```python
from build123d import *

# Parameters (mm, degrees)
PAD_DEPTH       = 15
PAD001_DEPTH    = 15
SKETCH002_R     = 4
POCKET_DEPTH    = 30
POCKET001_DEPTH = 4
SKETCH004_W     = 15
SKETCH004_H     = 50
PAD002_DEPTH    = 40
PAD003_DEPTH    = 50
SKETCH006_W     = 20
SKETCH006_H     = 5
POCKET002_DEPTH = 15
SKETCH007_W     = 30
SKETCH007_H     = 7.2
POCKET003_DEPTH = 3
SKETCH008_W     = 173.297394
SKETCH008_H     = 63.43742
POCKET004_DEPTH = 100
SKETCH009_W     = 20
SKETCH009_H     = 30
PAD004_DEPTH    = 15
SKETCH010_W     = 15
SKETCH010_H     = 30
PAD005_DEPTH    = 60
SKETCH011_R     = 2.5
POCKET005_DEPTH = 15
PAD006_DEPTH    = 30
SKETCH013_W     = 15
SKETCH013_H     = 20
POCKET006_DEPTH = 30
SKETCH014_R     = 2.5
POCKET007_DEPTH = 15
SKETCH015_R     = 6.7
POCKET008_DEPTH = 15
POCKET009_DEPTH = 4
SKETCH017_R     = 5.75
SKETCH017_R_2   = 4
PAD007_DEPTH    = 4
PAD008_DEPTH    = 15
SKETCH019_W     = 30
SKETCH019_H     = 12.5
POCKET010_DEPTH = 15
SKETCH020_R     = 2.5
POCKET011_DEPTH = 15


with BuildPart() as part:
    # Sketch → Pad (new body)
    with BuildSketch(Plane.XY):
        with BuildLine():
            ThreePointArc((6.422616, 1), (-6.5, 0), (6.422616, -1))
            Line((6.422616, -1), (20, -1))
            Line((20, -1), (20, -15))
            Line((20, -15), (-15, -15))
            Line((-15, -15), (-15, -7.5))
            Line((-30, -7.5), (-15, -7.5))
            Line((-45, -22.5), (-30, -7.5))
            Line((-45, -22.5), (-45, -45))
            Line((-180, -45), (-45, -45))
            Line((-180, 45), (-180, -45))
            Line((-180, 45), (-45, 45))
            Line((-45, 22.5), (-45, 45))
            Line((-45, 22.5), (-30, 7.5))
            Line((-30, 7.5), (-15, 7.5))
            Line((-15, 7.5), (-15, 15))
            Line((-15, 15), (20, 15))
            Line((20, 15), (20, 1))
            Line((6.422616, 1), (20, 1))
        make_face()
        Polygon((-60, 30), (-60, 2.330407), (-60, -7.217157), (-60, -30), (-165, -30), (-165, 30), align=None, mode=Mode.SUBTRACT)
    extrude(amount=PAD_DEPTH)

    # Sketch001 → Pad001 (new body)
    with BuildSketch(Plane.XY.offset(15)):
        Polygon((-165, 30), (-165, 20), (-150, 30), align=None)
        Polygon((-165, -20), (-165, -30), (-150, -30), align=None)
    extrude(amount=-PAD001_DEPTH)

    # Sketch002 → Pocket (cut)
    with BuildSketch(Plane.XZ.offset(15)):
        with Locations((10, 7.5)):
            Circle(SKETCH002_R)
    extrude(amount=-POCKET_DEPTH, mode=Mode.SUBTRACT)

    # Sketch003 → Pocket001 (cut)
    with BuildSketch(Plane.XZ.offset(15)):
        Polygon((12.875, 2.520354), (15.75, 7.5), (12.875, 12.479646), (7.125, 12.479646), (4.25, 7.5), (7.125, 2.520354), align=None)
    extrude(amount=-POCKET001_DEPTH, mode=Mode.SUBTRACT)

    # Sketch004 → Pad002 (new body)
    with BuildSketch(Plane.XY.offset(15)):
        with Locations((-172.5, 0)):
            Rectangle(SKETCH004_W, SKETCH004_H)
    extrude(amount=PAD002_DEPTH)

    # Sketch005 → Pad003 (new body)
    with BuildSketch(Plane(origin=(0, 25, 0), x_dir=(-1, 0, 0), z_dir=(0, 1, 0))):
        Polygon((180, 25), (190, 15), (190, 0), (180, 0), align=None)
    extrude(amount=-PAD003_DEPTH)

    # Sketch006 → Pocket002 (cut)
    with BuildSketch(Plane.YZ.offset(-165)):
        with Locations((0, 33.434408)):
            Rectangle(SKETCH006_W, SKETCH006_H)
    extrude(amount=-POCKET002_DEPTH, mode=Mode.SUBTRACT)

    # Sketch007 → Pocket003 (cut)
    with BuildSketch(Plane.YZ.offset(-165)):
        with Locations((0, 33.791532)):
            Rectangle(SKETCH007_W, SKETCH007_H)
    extrude(amount=-POCKET003_DEPTH, mode=Mode.SUBTRACT)

    # Sketch008 → Pocket004 (cut)
    with BuildSketch(Plane(origin=(0, 45, 0), x_dir=(-1, 0, 0), z_dir=(0, 1, 0))):
        with Locations((116.648697, 31.71871)):
            Rectangle(SKETCH008_W, SKETCH008_H)
    extrude(amount=-POCKET004_DEPTH, mode=Mode.SUBTRACT)

    # Sketch009 → Pad004 (new body)
    with BuildSketch(Plane.XY.offset(15)):
        with Locations((-25, 0)):
            Rectangle(SKETCH009_W, SKETCH009_H)
    extrude(amount=-PAD004_DEPTH)

    # Sketch010 → Pad005 (new body)
    with BuildSketch(Plane.XY.offset(15)):
        with Locations((-27.5, 0)):
            Rectangle(SKETCH010_W, SKETCH010_H)
    extrude(amount=PAD005_DEPTH)

    # Sketch011 → Pocket005 (cut)
    with BuildSketch(Plane.YZ.offset(-20)):
        with Locations((0, 65)):
            Circle(SKETCH011_R)
    extrude(amount=-POCKET005_DEPTH, mode=Mode.SUBTRACT)

    # Sketch012 → Pad006 (new body)
    with BuildSketch(Plane(origin=(0, 15, 0), x_dir=(-1, 0, 0), z_dir=(0, 1, 0))):
        Polygon((10, 15), (20, 25), (20, 15), align=None)
    extrude(amount=-PAD006_DEPTH)

    # Sketch013 → Pocket006 (cut)
    with BuildSketch(Plane.XZ.offset(15)):
        with Locations((-27.5, 65)):
            Rectangle(SKETCH013_W, SKETCH013_H)
    extrude(amount=-POCKET006_DEPTH, mode=Mode.SUBTRACT)

    # Sketch014 → Pocket007 (cut)
    with BuildSketch(Plane.YZ.offset(-20)):
        with Locations((0, 45)):
            Circle(SKETCH014_R)
    extrude(amount=-POCKET007_DEPTH, mode=Mode.SUBTRACT)

    # Sketch015 → Pocket008 (cut)
    with BuildSketch(Plane(origin=(0, 0, 0), x_dir=(1, 0, 0), z_dir=(0, 0, -1))):
        Circle(SKETCH015_R)
    extrude(amount=-POCKET008_DEPTH, mode=Mode.SUBTRACT)

    # Sketch016 → Pocket009 (cut)
    with BuildSketch(Plane(origin=(0, 15, 0), x_dir=(-1, 0, 0), z_dir=(0, 1, 0))):
        Polygon((-5.020354, 4.625), (-5.020354, 10.375), (-10, 13.25), (-14.979646, 10.375), (-14.979646, 4.625), (-10, 1.75), align=None)
    extrude(amount=-POCKET009_DEPTH, mode=Mode.SUBTRACT)

    # Sketch017 → Pad007 (new body)
    with BuildSketch(Plane.XZ.offset(15)):
        with Locations((10, 7.5)):
            Circle(SKETCH017_R)
        with Locations((10, 7.5)):
            Circle(SKETCH017_R_2, mode=Mode.SUBTRACT)
    extrude(amount=-PAD007_DEPTH)

    # Sketch018 → Pad008 (new body)
    with BuildSketch(Plane(origin=(0, 0, 0), x_dir=(1, 0, 0), z_dir=(0, 0, -1))):
        with BuildLine():
            ThreePointArc((6.523803, 1), (-6.6, 0), (6.523803, -1))
            Line((6.523803, -1), (6.726069, -1))
            ThreePointArc((6.726069, 1), (-6.8, 0), (6.726069, -1))
            Line((6.523803, 1), (6.726069, 1))
        make_face()
    extrude(amount=-PAD008_DEPTH)

    # Sketch019 → Pocket010 (cut)
    with BuildSketch(Plane.YZ.offset(-20)):
        with Locations((0, 48.75)):
            Rectangle(SKETCH019_W, SKETCH019_H)
    extrude(amount=-POCKET010_DEPTH, mode=Mode.SUBTRACT)

    # Sketch020 → Pocket011 (cut)
    with BuildSketch(Plane.YZ.offset(-20)):
        with Locations((0, 34.5)):
            Circle(SKETCH020_R)
    extrude(amount=-POCKET011_DEPTH, mode=Mode.SUBTRACT)


solid = part.part
```
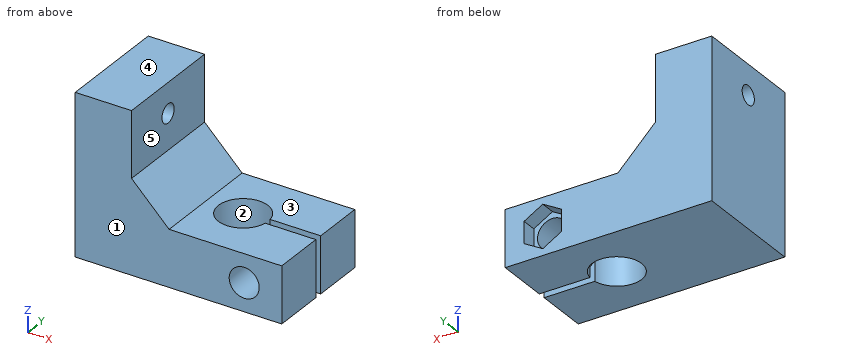
The listing builds one solid part. Answer for the finished solid, in the listing's coordinates (mm). Face numbers are marked on the shaded views. A direction names the side the tool comes from. Give positions to 0.01 mm unless a question says otherwise; leave off trailing zeros. Write each loop counter-clockwise with the first axis right and the second up, starting at its lowest first coordinate (ties: lowest second). Pieces come first, ordered by that corner, then holes. Notation, with made-up numbers: (15, -27) -> (29, -27) arc R25 cw to (29, -4) -> close; hole circle Ø2 at (-4, -14). An arc over 180 degrees is marked (long way). Use one line per item in the form item = value.
1) A tool of negligible diameter and unlimited length cuts with its end or side. For the marked faces 4 and 5, from which of +Z, -Z, +X, -X, +Y, -Y can it reach the whole face along a straight path? Write none if from no direction.
Result:
face_4 = +Z, +X, -X, +Y, -Y
face_5 = +Z, +X, +Y, -Y
2) Straight lines are drawn through the part: probe 1 along Y at (x, z) = (0, 10); probe 2 along Z at (x, y) = (-32, 0); probe 3 along X at (y, z) = (-4.75, 7.5). For each, find the intervals that lie inside material, in ascending order.
Result:
probe_1 = -15 to -6.6, 6.6 to 15
probe_2 = 0 to 32, 37 to 42.5
probe_3 = -35 to -4.58, 4.58 to 6, 14 to 20
3) Section C-C on z = 7.5 is taken. Write down the section's boundary in (x, y), plus the area to 3 significant figures.
Result:
outline = (-35, -15) -> (6, -15) -> (6, -3.2) arc R6.8 ccw to (6.73, -1) -> (6.52, -1) arc R6.6 cw (long way) to (6.52, 1) -> (6.73, 1) arc R6.8 ccw to (6, 3.2) -> (6, 11) -> (5.02, 11) -> (5.02, 15) -> (-35, 15) -> close; (14, -15) -> (20, -15) -> (20, -1) -> (14, -1) -> close; (14, 1) -> (20, 1) -> (20, 15) -> (14.98, 15) -> (14.98, 11) -> (14, 11) -> close
area = 1,260 mm²
4) Each of these flat-tipped pins is pushed along its axis until it touches: P1, Ø8, axis at x = 11.5, z = 9.5, coming from the +Y side; P2, Ø10, axis at x = 4, y = 3.5, coming from the +Z side; P3, Ø8, axis at y = 0, z = 34.5, coming from the +X side. Where does it stop, or does it pass through?
Result:
P1 = 15
P2 = 15
P3 = -20
5) Section B-B on z = 34.5 is taken. Write down the section's boundary in (x, y), plus the area to 3 significant figures.
Result:
outline = (-35, -15) -> (-20, -15) -> (-20, -2.5) -> (-35, -2.5) -> close; (-35, 2.5) -> (-20, 2.5) -> (-20, 15) -> (-35, 15) -> close
area = 375 mm²
6) Section A-A on x = 0 is taken. Write down the section's boundary in (y, z), plus the area to 3 significant figures.
Result:
outline = (-15, 0) -> (-6.6, 0) -> (-6.6, 15) -> (-15, 15) -> close; (6.6, 0) -> (15, 0) -> (15, 15) -> (6.6, 15) -> close
area = 252 mm²
7) For a pull along Y with two mould halves and no side action, classify the marked faces 1, 2 and 3 as +Y half, -Y half, draft (parallel to the pull), parting line (faces both ways), or undercut.
Result:
face_1 = -Y half
face_2 = undercut
face_3 = draft
8) Section D-D on y = -9 is taken. Write down the section's boundary in (x, z).
Result:
outline = (-35, 0) -> (20, 0) -> (20, 15) -> (-10, 15) -> (-20, 25) -> (-20, 42.5) -> (-35, 42.5) -> close; hole circle Ø8 at (10, 7.5)
